Geometry: final body of the model. Coordinates: model frame, mm. A direction names the side the tool comes from. Give positions to 0.01 mm unless a question says otherwise; leave off trailing zeros. Write each loop counter-clockwise with the first axis right and the second up, starting at its lowest first coordinate (ties: lowest second). Pieces come first, ordered by that corner, then holes. Notation, with made-up numbers: (74.5, -11.5) - (106.5, -11.5) arc R34 ccw to (106.5, 27.5) - close; hole circle Ø2 at (14.5, 28.5). An arc over 180 degrees is marked (long way). Return JSON: item names as keys, results as strings.
from build123d import *

# Parameters (mm, degrees)
F1_DEPTH = 60
F2_R     = 4.125
F2_R_2   = 3.996282
F2_R_3   = 4.670247
F3_DEPTH = 5
F4_R     = 4
F5_DEPTH = 50.001


with BuildPart() as f1:
    # F0 (on Front) → F1 (new body)
    with BuildSketch(Plane.XZ):
        Polygon((-20, 18.727273), (-20, 0), (20, 0), (20, 18.727273), (10, 18.727273), (10, 8.727273), (-10, 8.727273), (-10, 18.727273), align=None)
    extrude(amount=F1_DEPTH)

    # F2 (on face) → F3 (join)
    with BuildSketch(Plane.XZ.offset(60)):
        with BuildLine():
            Line((20, 50), (-20, 50))
            ThreePointArc((-20, 50), (-30.606602, 45.606602), (-35, 35))
            Line((-35, 35), (-35, -15))
            ThreePointArc((-35, -15), (-30.606602, -25.606602), (-20, -30))
            Line((-20, -30), (20, -30))
            ThreePointArc((20, -30), (30.606602, -25.606602), (35, -15))
            Line((35, -15), (35, 35))
            ThreePointArc((35, 35), (30.606602, 45.606602), (20, 50))
        make_face()
        with Locations((-20, -15)):
            Circle(F2_R, mode=Mode.SUBTRACT)
        with Locations((20, -15)):
            Circle(F2_R_2, mode=Mode.SUBTRACT)
        with Locations((-20, 35)):
            Circle(F2_R, mode=Mode.SUBTRACT)
        with Locations((20, 35)):
            Circle(F2_R_3, mode=Mode.SUBTRACT)
    extrude(amount=F3_DEPTH)

    # F4 (on Top) → F5 (cut, through all)
    with BuildSketch(Plane.XY):
        with Locations((0, -49)):
            Circle(F4_R)
        with Locations((0, -24)):
            Circle(F4_R)
    extrude(amount=F5_DEPTH, mode=Mode.SUBTRACT)


solid = f1.part
Q1. Set-up query: faces 5 (the flat face through (0, -30, 0)), 6 (the cylindrical face through (30.49, -62.46, -25.72)), 7 (the flat face through (0, -30, 8.727)), 8 (the flat face through (20, -30, 9)). Return all of +Z, -Z, +X, -X, +Y, -Y with unobstructed straight access to the full face (end or side cutting, diameter ignored); none if empty.
Answer key:
{"face 5": "-Z, +X, -X, +Y", "face 6": "-Z, +X, +Y, -Y", "face 7": "+Z, +Y", "face 8": "+Z, -Z, +X, +Y"}
Q2. Section query D-D, the plane y = -34. Return the cut outline in (x, z), plus the area to 3 significant figures.
Answer key:
{"outline": "(-20, 0) - (20, 0) - (20, 18.73) - (10, 18.73) - (10, 8.73) - (-10, 8.73) - (-10, 18.73) - (-20, 18.73) - close", "area": "549 mm^2"}
Q3. Material intervals for probe 1 along Z at (x, y) = (20, -62.5); probe 2 along Y at (x, z) = (0, 5); probe 3 along Z at (x, y) = (-20, -64) (3 decimals), sorted ascending. Write a range as [from, to].
Answer key:
{"probe 1": "z = [-30, -19], [-11, 30.33], [39.67, 50]", "probe 2": "y = [-65, -53], [-45, -28], [-20, 0]", "probe 3": "z = [-30, -19.125], [-10.875, 30.875], [39.125, 50]"}
Q4. Section query A-A, the plane y = -24. Return the cut outline in (x, z), plus the area to 3 significant figures.
Answer key:
{"outline": "(-20, 0) - (-4, 0) - (-4, 8.73) - (-10, 8.73) - (-10, 18.73) - (-20, 18.73) - close; (4, 0) - (20, 0) - (20, 18.73) - (10, 18.73) - (10, 8.73) - (4, 8.73) - close", "area": "479 mm^2"}
Q5. Pin query (flat end, axial travel): P1, Ø6.5, axis at x = -20, z = 35, coming from the +Y side; P2, Ø10, axis at x = 4.5, z = 23, coming from the +Y side; P3, Ø5, axis at x = -16.5, y = -23.5, coming from the +Z side; P4, Ø2, axis at x = 12, z = 0.5, coming from the +Y side. Return the tip coordinate at first contact, or that it passes through.
Answer key:
{"P1": "passes through", "P2": "stops at y = -60", "P3": "stops at z = 18.73", "P4": "stops at y = 0"}
Q6. Mould query, pull axis Z, two halves, no side actions, for faces 1 (the flat face through (15, -30, 18.727)), 2 (the cylindrical face through (-23.273, -62.465, 32.49)), 3 (the cylindrical face through (1.846, -52.549, 4.303)), 4 (the cylindrical face through (16.008, -62.465, -14.824)). Classes: pulls with the +Z half, pulls with the -Z half, needs draft (parallel to the pull), parting line crosses it, or undercut.
Answer key:
{"face 1": "pulls with the +Z half", "face 2": "undercut", "face 3": "needs draft", "face 4": "undercut"}
Q7. Section query C-C, the plane z = 16.5. Return the cut outline in (x, y), plus the area to 3 significant figures.
Answer key:
{"outline": "(-35, -65) - (35, -65) - (35, -60) - (20, -60) - (20, 0) - (10, 0) - (10, -60) - (-10, -60) - (-10, 0) - (-20, 0) - (-20, -60) - (-35, -60) - close", "area": "1,550 mm^2"}
Q8. Section query B-B, the plane x = 0. Return the cut outline in (y, z), plus the area to 3 significant figures.
Answer key:
{"outline": "(-65, -30) - (-60, -30) - (-60, 0) - (-53, 0) - (-53, 8.73) - (-60, 8.73) - (-60, 50) - (-65, 50) - close; (-45, 0) - (-28, 0) - (-28, 8.73) - (-45, 8.73) - close; (-20, 0) - (0, 0) - (0, 8.73) - (-20, 8.73) - close", "area": "784 mm^2"}
